Model file for the job. Use its own axes, mm. Face numbers are marked on the shaded views. A direction names the side the tool comes from. Give positions to 0.01 mm unless a question says otherwise; leave off trailing zeros. Order: outer loops, then holes, each group sorted by start corner. A loop starts at its lowest first (then second) coordinate and runs counter-clockwise, first axis right, second up. Notation, with made-up numbers: M 1.5,-24 L 12.5,-24 A14 ccw 12.5,1 Z; hole C 28,68 d1. An arc over 180 degrees is marked long. Return JSON: item names as keys, results as strings. Group by question number.
1. Slice it at B-B on z = -23.4. List the corners of the cut face in (x, y).
2. Slice it at A-A on x = 0. List the corners of the cut face in (y, z), then the cut area to 3 significant figures.
3. 3-axis set-ups, long thin cutter, end or side, ignore diameter. For the marked faces 1 and 2: which of +Z, -Z, +X, -X, +Y, -Y reach the whole face in a straight line?
4. Two-plate mould, pull along Y, no slides. Class the marked faces 3, 4 and 5: released by +Y, released by -Y, zero draft, split by the parting line, or undercut.
5. Pin check, flat tips, straight feed: pin 1 (1 mm diameter, centred on y = 27, z = -3.5, fed in from +X); pin 2 (8 mm diameter, centred on y = 42, z = -26.5, fed in from -X); pin 3 (6 mm diameter, centred on y = 17, z = -4, fed in from +X); pin 4 (6 mm diameter, centred on x = -26.5, z = -18.5, fed in from -Y). Stop position of each tip, or through.
6. Wall check: probe 1 along X at (y, z) = (48.85, -23.4); probe 2 along Y at (x, z) = (0, -7); probe 3 along Z at (x, y) = (30, 56.15). Give the ranges that are in metal, low to high. Write a range as [from, to].
from build123d import *

# Parameters (mm, degrees)
BASE_EXTRUDE_DEPTH      = 38
CUT_EXTRUDE1_DEPTH      = 81.554329493
CUT_EXTRUDE1_DEPTH_BACK = 41
HOLE2_OUTLINE_R         = 11
HOLE2_DEPTH             = 2
HOLE2_START             = -10
HOLE2_2_OUTLINE_R       = 11
HOLE2_2_DEPTH           = 10
HOLE2_START_2           = 48
HOLE2_3_OUTLINE_R       = 10
HOLE2_3_DEPTH           = 4
HOLE2_START_3           = 52
HOLE2_4_OUTLINE_R       = 5.5
HOLE2_4_DEPTH           = 6
FILLET1_R               = 10
FILLET7_R               = 1.5


with BuildPart() as part:
    # Sketch2 → Base-Extrude (new body)
    with BuildSketch(Plane.XY):
        with BuildLine():
            Line((-14.402593128, -6.96888163), (-41, 48))
            Line((-41, 48), (-41, 58))
            Line((-41, 58), (41, 58))
            Line((41, 58), (41, 48))
            Line((41, 48), (14.402593128, -6.96888163))
            ThreePointArc((14.402593128, -6.96888163), (0, -16), (-14.402593128, -6.96888163))
        make_face()
    extrude(amount=-BASE_EXTRUDE_DEPTH)

    # Sketch3 → Cut-Extrude1 (cut, two sides: drawn at the far end of the back side and taken through both)
    with BuildSketch(Plane(origin=(0, 0, 0), x_dir=(0, 0, -1), z_dir=(1, 0, 0)).offset(-CUT_EXTRUDE1_DEPTH_BACK)):
        Polygon((10, -250.492798217), (10, -38.853504021), (10, 48), (38, 48), (249.639294197, 48), (579.708021452, -216.989431263), (340.068727255, -515.482229481), align=None)
    extrude(amount=CUT_EXTRUDE1_DEPTH + CUT_EXTRUDE1_DEPTH_BACK, mode=Mode.SUBTRACT)

    # Hole2: read off the stored shape, not the designer's step
    # Hole2 outline → Hole2 (add)
    with BuildSketch(Plane.XY):
        with BuildLine():
            ThreePointArc((14.402593128, -6.96888163), (0, 16), (-14.402593128, -6.96888163))
            ThreePointArc((-14.402593128, -6.96888163), (0, -16), (14.402593128, -6.96888163))
        make_face()
        Circle(HOLE2_OUTLINE_R, mode=Mode.SUBTRACT)
    hole2 = extrude(amount=HOLE2_DEPTH)

    # Hole2 2 outline → Hole2 2 (cut)
    with BuildSketch(Plane.XY.offset(HOLE2_START)):
        Circle(HOLE2_2_OUTLINE_R)
    hole2_2 = extrude(amount=HOLE2_2_DEPTH, mode=Mode.SUBTRACT)

    # Hole2 3 outline → Hole2 3 (cut)
    with BuildSketch(Plane(origin=(0, 0, 0), x_dir=(1, 0, 0), z_dir=(0, 1, 0)).offset(HOLE2_START_2)):
        with Locations((30, 23.4)):
            Circle(HOLE2_3_OUTLINE_R)
    hole2_3 = extrude(amount=HOLE2_3_DEPTH, mode=Mode.SUBTRACT)

    # Hole2 4 outline → Hole2 4 (cut)
    with BuildSketch(Plane(origin=(0, 0, 0), x_dir=(1, 0, 0), z_dir=(0, 1, 0)).offset(HOLE2_START_3)):
        with Locations((30, 23.4)):
            Circle(HOLE2_4_OUTLINE_R)
    hole2_4 = extrude(amount=HOLE2_4_DEPTH, mode=Mode.SUBTRACT)

    # Mirror1: Hole2, Hole2 2, Hole2 3, Hole2 4 across plane
    add(hole2.mirror(Plane(origin=(0, 0, 0), x_dir=(0, 0, 1), z_dir=(1, 0, 0))))
    add(hole2_2.mirror(Plane(origin=(0, 0, 0), x_dir=(0, 0, 1), z_dir=(1, 0, 0))), mode=Mode.SUBTRACT)
    add(hole2_3.mirror(Plane(origin=(0, 0, 0), x_dir=(0, 0, 1), z_dir=(1, 0, 0))), mode=Mode.SUBTRACT)
    add(hole2_4.mirror(Plane(origin=(0, 0, 0), x_dir=(0, 0, 1), z_dir=(1, 0, 0))), mode=Mode.SUBTRACT)

    # Fillet1
    fillet1_edges = [part.edges().sort_by_distance(p)[0] for p in [
        (41, 53, -38),
        (-41, 53, -38),
    ]]
    fillet(fillet1_edges, radius=FILLET1_R)

    # Fillet7
    # the kernel refuses this fillet: 1.5 mm, written as the material it takes off along each edge
    with BuildSketch(Plane(origin=(14.402593128, -6.96888163, -10), x_dir=(-0.9001620705215131, 0.43555510190379193, 0), z_dir=(0.435555101903792, 0.9001620705215131, 0))) as fillet7_piece_1_section:
        with BuildLine():
            CenterArc((FILLET7_R, FILLET7_R), FILLET7_R, 180, 90)
            Line((0, FILLET7_R), (0, 0))
            Line((0, 0), (FILLET7_R, 0))
        make_face()
    fillet7_piece_1 = extrude(amount=64.815538563, mode=Mode.PRIVATE)
    fillet7_piece_1 = split(fillet7_piece_1, bisect_by=Plane(origin=(14.402593128, 48, -10), z_dir=(0, -1, 0)), keep=Keep.TOP, mode=Mode.PRIVATE)
    add(fillet7_piece_1, mode=Mode.SUBTRACT)
    with BuildSketch(Plane(origin=(0, 0, -10), x_dir=(-0.9001620705215129, -0.4355551019037922, 0), z_dir=(-0.4355551019037922, 0.9001620705215129, 0))) as fillet7_piece_2:
        with BuildLine():
            CenterArc((16 - FILLET7_R, FILLET7_R), FILLET7_R, 270, 90)
            Line((16, FILLET7_R), (16, 0))
            Line((16, 0), (16 - FILLET7_R, 0))
        make_face()
    revolve(axis=Axis((0, 0, -10), (0, 0, 1)), revolution_arc=128.358757734, mode=Mode.SUBTRACT)
    with BuildSketch(Plane(origin=(-42.633331632, 51.375607764, -10), x_dir=(0, 0, 1), z_dir=(0.4355551019037922, -0.900162070521513, 0))) as fillet7_piece_3_section:
        with BuildLine():
            CenterArc((FILLET7_R, -FILLET7_R), FILLET7_R, 90, 90)
            Line((0, -FILLET7_R), (0, 0))
            Line((0, 0), (FILLET7_R, 0))
        make_face()
    fillet7_piece_3 = extrude(amount=64.815538563, mode=Mode.PRIVATE)
    fillet7_piece_3 = split(fillet7_piece_3, bisect_by=Plane(origin=(-42.633331632, 48, -10), z_dir=(0, -1, 0)), keep=Keep.TOP, mode=Mode.PRIVATE)
    add(fillet7_piece_3, mode=Mode.SUBTRACT)
    with BuildSketch(Plane(origin=(-31, 58, -38), x_dir=(0, 0, 1), z_dir=(1, 0, 0))) as fillet7_piece_4:
        with BuildLine():
            CenterArc((FILLET7_R, FILLET7_R), FILLET7_R, 180, 90)
            Line((0, FILLET7_R), (0, 0))
            Line((0, 0), (FILLET7_R, 0))
        make_face()
    extrude(amount=62, mode=Mode.SUBTRACT)
    with BuildSketch(Plane(origin=(41, 58, 3.75), x_dir=(-1, 0, 0), z_dir=(0, 0, -1)), Plane(origin=(-41, 58, 3.75), x_dir=(0, -1, 0), z_dir=(0, 0, -1))) as fillet7_piece_5:
        with BuildLine():
            CenterArc((FILLET7_R, -FILLET7_R), FILLET7_R, 90, 90)
            Line((0, -FILLET7_R), (0, 0))
            Line((0, 0), (FILLET7_R, 0))
        make_face()
    extrude(amount=31.75, mode=Mode.SUBTRACT)
    with BuildSketch(Plane(origin=(31, 58, -28), x_dir=(1, 0, 0), z_dir=(0, 0, 1))) as fillet7_piece_6:
        with BuildLine():
            CenterArc((10 - FILLET7_R, -FILLET7_R), FILLET7_R, 360, 90)
            Line((10, -FILLET7_R), (10, 0))
            Line((10, 0), (10 - FILLET7_R, 0))
        make_face()
    revolve(axis=Axis((31, 58, -28), (0, 1, 0)), revolution_arc=90, mode=Mode.SUBTRACT)
    with BuildSketch(Plane(origin=(-31, 58, -28), x_dir=(-1, 0, 0), z_dir=(0, 0, 1))) as fillet7_piece_7:
        with BuildLine():
            CenterArc((10 - FILLET7_R, FILLET7_R), FILLET7_R, 270, 90)
            Line((10 - FILLET7_R, 0), (10, 0))
            Line((10, 0), (10, FILLET7_R))
        make_face()
    revolve(axis=Axis((-31, 58, -28), (0, -1, 0)), revolution_arc=90, mode=Mode.SUBTRACT)
    with BuildSketch(Plane(origin=(-9.502598232, -17.095704924, 0), x_dir=(0, 0, -1), z_dir=(-0.4355551019037922, 0.900162070521513, 0))) as fillet7_piece_8_section:
        with BuildLine():
            CenterArc((FILLET7_R, -FILLET7_R), FILLET7_R, 90, 90)
            Line((0, -FILLET7_R), (0, 0))
            Line((0, 0), (FILLET7_R, 0))
        make_face()
    fillet7_piece_8 = extrude(amount=76.065538563, mode=Mode.PRIVATE)
    fillet7_piece_8 = fillet7_piece_8 - Plane(origin=(0, 0, 0), x_dir=(0.9001620705200065, -0.4355551019069058, 0), z_dir=(0, 0, -1)) * Cylinder(16, 159, mode=Mode.PRIVATE)
    add(fillet7_piece_8, mode=Mode.SUBTRACT)
    with BuildSketch(Plane(origin=(-44.75, 58, 0), x_dir=(0, 0, -1), z_dir=(1, 0, 0))) as fillet7_piece_9:
        with BuildLine():
            CenterArc((FILLET7_R, -FILLET7_R), FILLET7_R, 90, 90)
            Line((0, -FILLET7_R), (0, 0))
            Line((0, 0), (FILLET7_R, 0))
        make_face()
    extrude(amount=89.5, mode=Mode.SUBTRACT)
    with BuildSketch(Plane(origin=(42.633331632, 51.375607764, 0), x_dir=(-0.900162070521513, 0.4355551019037919, 0), z_dir=(-0.435555101903792, -0.9001620705215131, 0))) as fillet7_piece_10_section:
        with BuildLine():
            CenterArc((FILLET7_R, FILLET7_R), FILLET7_R, 180, 90)
            Line((0, FILLET7_R), (0, 0))
            Line((0, 0), (FILLET7_R, 0))
        make_face()
    fillet7_piece_10 = extrude(amount=76.065538563, mode=Mode.PRIVATE)
    fillet7_piece_10 = fillet7_piece_10 - Plane(origin=(0, 0, 0), x_dir=(0.9001620705200065, -0.4355551019069058, 0), z_dir=(0, 0, -1)) * Cylinder(16, 159, mode=Mode.PRIVATE)
    add(fillet7_piece_10, mode=Mode.SUBTRACT)


solid = part.part
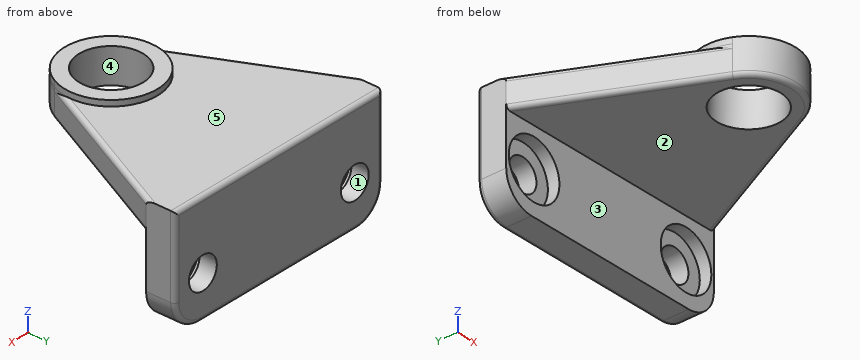
Result:
{
 "1": {"outline": "M -41,48 L -40,48 L -40,52 L -35.5,52 L -35.5,58 L -39.5,58 A1.5 ccw -41,56.5 Z; M -24.5,52 L -20,52 L -20,48 L 20,48 L 20,52 L 24.5,52 L 24.5,58 L -24.5,58 Z; M 35.5,52 L 40,52 L 40,48 L 41,48 L 41,56.5 A1.5 ccw 39.5,58 L 35.5,58 Z"},
 "2": {"outline": "M -16,-8.5 A1.5 ccw -14.5,-10 L -11,-10 L -11,2 L -16,2 Z; M 11,-10 L 48,-10 L 48,-38 L 56.5,-38 A1.5 ccw 58,-36.5 L 58,-1.5 A1.5 ccw 56.5,0 L 16,0 L 16,2 L 11,2 Z", "area": "819 mm2"},
 "3": {"face 1": "+Y, -Y", "face 2": "-Z, +X, -X, -Y"},
 "4": {"face 3": "released by -Y", "face 4": "undercut", "face 5": "zero draft"},
 "5": {"pin 1": "stops at x = 31.08", "pin 2": "passes through", "pin 3": "stops at x = 27.45", "pin 4": "stops at y = 52"},
 "6": {"probe 1": "x = [-41, -40], [-20, 20], [40, 41]", "probe 2": "y = [-16, -11], [11, 58]", "probe 3": "z = [-38, -28.9], [-17.9, 0]"}
}
